Read the model definition and answer for the solid it produces. Units are mm, in the model's axes. A direction names the side the tool comes from. Round coordinates to 2 decimals unless told otherwise and drop trailing zeros. Loops run counter-clockwise (first coordinate to the right, second up) from the corner with the lowest first, then second, coordinate; pieces in that order, holes last. Notation, with made-up numbers: (-28, 14.25) - (8, 14.25) arc R25 cw to (8, 26.25) - close; hole circle Ø7 at (18.5, 25). An arc over 180 degrees is marked (long way). Use one line per item in the form item = value. Start each with the question number.
```python
from build123d import *

# Parameters (mm, degrees)
F0_W         = 71
F0_H         = 145
F1_DEPTH     = 2
F2_W         = 7
F2_H         = 145
F3_DEPTH     = 8
F4_T         = 2
F5_W         = 3.7458891392
F5_H         = 131.9372802973
F6_DEPTH     = 2
F7_W         = 3.5460759103
F7_H         = 131.9372802973
F8_DEPTH     = 2
F9_R         = 5
F11_DEPTH    = 2.5
F13_DEPTH    = 2
F15_T1_DEPTH = 9.5
F15_T3_DEPTH = 10.6171437222
F15_T5_DEPTH = 10.816956951
F16_R        = 1
F14_W        = 10
F14_H        = 20
F17_DEPTH    = 2


# Not quite as in the source:
# - a fillet or chamfer that OpenCascade refuses, or shapes differently, is made with other operations: its cross-section is extruded or revolved along the edge and cut away or added
# - a shell that OpenCascade refuses in one call is made with other operations: the cavity is built on its own and cut out
# - a feature names something its author has since deleted; it is built from what else it names


with BuildPart() as f1:
    # F0 (on Front) → F1 (new body)
    with BuildSketch(Plane.XZ):
        Rectangle(F0_W, F0_H)
    extrude(amount=F1_DEPTH)

    # F2 (on face) → F3 (join)
    with BuildSketch(Plane.XZ.offset(2)):
        with Locations((-32, 0)):
            Rectangle(F2_W, F2_H)
        with Locations((32, 0)):
            Rectangle(F2_W, F2_H)
    extrude(amount=F3_DEPTH)

    # F4: shell of thickness 2, made by hand


with BuildPart() as f4_core1:
    # F4_t2: copy of F1
    add(f1.part)

    # the walls: a layer under each face that stays
    f4_faces = [f4_core1.faces().sort_by_distance(p)[0] for p in [
        (23.6666666667, -1.6666666667, 72.5),
        (0, 0, 0),
        (-23.6666666667, -1.6666666667, -72.5),
        (-35.5, -5, 0),
        (-32, -10, 0),
        (0, -2, 0),
        (32, -10, 0),
        (35.5, -5, 0),
    ]]
    thicken(f4_faces, amount=-F4_T, mode=Mode.SUBTRACT)


with BuildPart() as f1_1:
    add(f1.part)

    # what is left inside the walls is the cavity
    f4_cavity = [f4_core1.part.solids().sort_by_distance(p)[0] for p in [
        (33.48, -6, 0),
        (-28.52, -6, 0),
    ]]
    add(f4_cavity, mode=Mode.SUBTRACT)

    # F5 (on face) → F6 (cut)
    with BuildSketch(Plane.XZ.offset(10)):
        with Locations((-30.3729445696, 0.5088895559)):
            Rectangle(F5_W, F5_H)
    extrude(amount=-F6_DEPTH, mode=Mode.SUBTRACT)

    # F7 (on face) → F8 (cut)
    with BuildSketch(Plane.XZ.offset(10)):
        with Locations((30.2730379552, -1.6313598514)):
            Rectangle(F7_W, F7_H)
    extrude(amount=-F8_DEPTH, mode=Mode.SUBTRACT)

    # F9
    f9_edges = [f1_1.edges().sort_by_distance(p)[0] for p in [
        (-35.5, -5, 72.5),
        (35.5, -5, 72.5),
        (35.5, -5, -72.5),
        (-35.5, -5, -72.5),
    ]]
    fillet(f9_edges, radius=F9_R)

    # F10 (on face) → F11 (cut)
    with BuildSketch(Plane.XZ.offset(2)):
        with BuildLine():
            ThreePointArc((28.5, 62.2240006924), (27.0355339059, 65.7595345983), (23.5, 67.2240006924))
            Line((23.5, 67.2240006924), (3.5, 67.2240006924))
            Line((3.5, 67.2240006924), (3.5, 62.2240006924))
            ThreePointArc((3.5, 62.2240006924), (4.9644660941, 58.6884667864), (8.5, 57.2240006924))
            Line((8.5, 57.2240006924), (28.5, 57.2240006924))
            Line((28.5, 57.2240006924), (28.5, 62.2240006924))
        make_face()
    extrude(amount=-F11_DEPTH, mode=Mode.SUBTRACT)

    # F12 (on face) → F13 (cut)
    with BuildSketch(Plane(origin=(-35.5, 0, 0), x_dir=(0, -1, 0), z_dir=(-1, 0, 0))):
        Polygon((10, 52.5), (0, 52.5), (0, 12.5), (10, 12.5), (10, 47.0733729486), align=None)
    extrude(amount=-F13_DEPTH, mode=Mode.SUBTRACT)

    # F15: fillet of radius 3 on 4 edges, made by hand

    # F15_s2 → F15_t1 (cut)
    with BuildSketch(Plane.XZ.offset(8)):
        with BuildLine():
            ThreePointArc((28.5, 67.3372802973), (29.3786796564, 65.2159599537), (31.5, 64.3372802973))
            Line((31.5, 64.3372802973), (28.5, 64.3372802973))
            Line((28.5, 64.3372802973), (28.5, 67.3372802973))
        make_face()
        with BuildLine():
            ThreePointArc((-28.5, 69.4775297046), (-29.3786796564, 67.356209361), (-31.5, 66.4775297046))
            Line((-31.5, 66.4775297046), (-28.5, 66.4775297046))
            Line((-28.5, 66.4775297046), (-28.5, 69.4775297046))
        make_face()
    extrude(amount=F15_T1_DEPTH, mode=Mode.SUBTRACT)

    # F15_s4 → F15_t3 (cut)
    with BuildSketch(Plane.YZ.offset(21.4289321881)):
        with BuildLine():
            ThreePointArc((-10, -67.6), (-8.5505102572, -68.6963763172), (-8, -70.4284271247))
            Line((-8, -70.4284271247), (-8, -67.6))
            Line((-8, -67.6), (-10, -67.6))
        make_face()
    extrude(amount=F15_T3_DEPTH, mode=Mode.SUBTRACT)

    # F15_s6 → F15_t5 (cut)
    with BuildSketch(Plane.YZ.offset(-32.2458891392)):
        with BuildLine():
            ThreePointArc((-8, -68.2881777175), (-8.5505102572, -66.5561269099), (-10, -65.4597505927))
            Line((-10, -65.4597505927), (-8, -65.4597505927))
            Line((-8, -65.4597505927), (-8, -68.2881777175))
        make_face()
    extrude(amount=F15_T5_DEPTH, mode=Mode.SUBTRACT)

    # F16
    f16_edges = [f1_1.edges().sort_by_distance(p)[0] for p in [
        (33.5, -5, 70.5),
        (-33.5, -5, 70.5),
        (-33.5, -5, -70.5),
        (33.5, -5, -70.5),
    ]]
    fillet(f16_edges, radius=F16_R)

    # F14 (on face) → F17 (cut)
    with BuildSketch(Plane.YZ.offset(35.5)):
        with Locations((-5, 42.1337091768)):
            Rectangle(F14_W, F14_H)
    extrude(amount=-F17_DEPTH, mode=Mode.SUBTRACT)


solid = f1_1.part
```
1) A cutting plane is placed at D-D on z = 39. Write down the section's boundary in (x, y).
2) A cutting plane is placed at A-A on z = 20. Write down the section's boundary in (x, y), plus the area to 3 significant figures.
3) Straight lines are drawn through the part: line 1 (X direction, y = -7, z = 66); line 2 (Z direction, x = -29, y = -4.25); line 3 (Y direction, x = -21.5, z = -3.5). For each, find the intervals that lie inside material, in ascending order. Write a range as from..to.
4) Flat-ended cylindrical pins translate along their axes: pin 1 (1 mm diameter, centred on y = -1, z = 40.5, fed in from -X); pin 2 (1.5 mm diameter, centred on y = -5, z = 70.5, fed in from -X); pin 3 (0.9 mm diameter, centred on y = -5.5, z = 71, fed in from +X). Find the tip coordinate at first contact, or state that the pin passes through.
5) A cutting plane is placed at B-B on y = -6.25. Count the separate pieces of the cut face and the enclosed holes in it, plus the area to 3 significant figures.
6) Determine the mould class of faces 5 (the flat face through (33.5, -5, -19)), 6 (the flat face through (0, -1, 72.5)), 7 (the flat face through (35.5, -5, -18)) for opening direction X: +X half, -X half, draft (parallel to the pull), parting line (faces both ways), or undercut.
7) A cutting plane is placed at C-C on x = 27. Write down the section's boundary in (y, z), plus the area to 3 significant figures.
8) For faces 1 (the cylindrical face through (30.248, -8.566, -68.675)), 2 (the flat face through (-28.5, -7, -71)), 3 (the cylindrical face through (27.074, -1.014, 65.72)), 4 (the flat face through (0, -1, -72.5)), determine the directions among +Z, -Z, +X, -X, +Y, -Y from which every point of the face is accessible in a straight line to the end or side of a thin tool.
Checks:
q1.outline = (-33.5, -10) - (-32.25, -10) - (-32.25, -8) - (-33.5, -8) - close; (-33.5, -2) - (33.5, -2) - (33.5, 0) - (-33.5, 0) - close; (32.05, -10) - (33.5, -10) - (33.5, -8) - (32.05, -8) - close
q2.outline = (-33.5, -10) - (-32.25, -10) - (-32.25, -8) - (-33.5, -8) - close; (-33.5, -2) - (33.5, -2) - (33.5, -8) - (32.05, -8) - (32.05, -10) - (35.5, -10) - (35.5, 0) - (-33.5, 0) - close
q2.area = 159 mm²
q3.line_1 = -35.5..-33.5, 33.5..35.5
q3.line_2 = -72.5..-70.5, 70.5..72.5
q3.line_3 = -2..0
q4.pin_1 = -33.5
q4.pin_2 = -34.97
q4.pin_3 = 34.46
q5.separate_pieces = 4
q5.enclosed_holes = 0
q5.area = 479 mm²
q6.face_5 = undercut
q6.face_6 = draft
q6.face_7 = +X half
q7.outline = (-2, -72.5) - (0, -72.5) - (0, 57.22) - (-2, 57.22) - close; (-2, 65.79) - (0, 65.79) - (0, 72.5) - (-2, 72.5) - close
q7.area = 273 mm²
q8.face_1 = none
q8.face_2 = +Z, -Z, -Y
q8.face_3 = +Y, -Y
q8.face_4 = -Z, +X, -X, +Y, -Y
